Check sheet for the modelled part. Datum: model origin and axes. Units: mm. Coordinates: 2 decimals unless noted, no trailing zeros. Loops run counter-clockwise (first coordinate to the right, second up) from the corner with the lowest first, then second, coordinate; pieces in that order, holes last. Notation, with made-up numbers: (28.25, -13) -> (57.25, -13) arc R10 ccw to (57.25, 0) -> close; hole circle Ø9 at (19, -30). An arc over 180 degrees is marked (long way). Use CSV: the item, a comma, the result in double quotes.
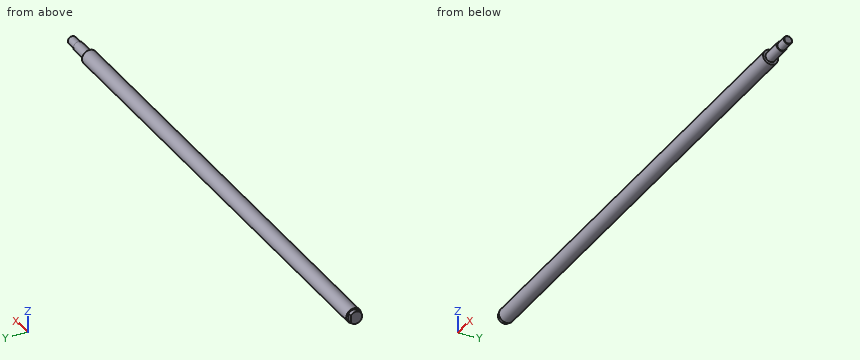
```python
from build123d import *

# Parameters (mm, degrees)
CHAMFER1_SIZE       = 0.5
BOSS_EXTRUDE1_DEPTH = 5


with BuildPart() as part:
    # Sketch1 → Revolve1 (revolve)
    with BuildSketch(Plane.XY, mode=Mode.PRIVATE) as revolve1_sk:
        Polygon((0, 0), (-640, 0), (-640, 9), (-40, 9), (-40, 6), (-15, 6), (-15, 5), (0, 5), align=None)
    revolve(revolve1_sk.sketch.rotate(Axis((-640, 0, 0), (1, 0, 0)), 90), axis=Axis((-640, 0, 0), (1, 0, 0)))

    # Chamfer1
    chamfer1_edges = [part.edges().sort_by_distance(p)[0] for p in [
        (0, 0, -5),
    ]]
    chamfer(chamfer1_edges, length=CHAMFER1_SIZE)

    # Sketch2 → Boss-Extrude1 (add)
    with BuildSketch(Plane.ZY.offset(640)):
        with BuildLine():
            Line((-4.485716723, 6.010685941), (4.485716723, 6.010685941))
            ThreePointArc((4.485716723, 6.010685941), (0, -7.5), (-4.485716723, 6.010685941))
        make_face()
    extrude(amount=BOSS_EXTRUDE1_DEPTH)


solid = part.part
```
1) Go/stop test with flat-tipped pins: pin 1 Ø8 at (x, z) = (-353, 2.5) entering from +Y; pin 2 Ø1.5 at (x, z) = (-355, 3.5) entering from +Y; pin 3 Ø5 at (y, z) = (-7, -3) entering from +X; pin 4 Ø6 at (x, z) = (-177.5, -7) entering from +Y. Record where each tip stops, or that it passes through.
Answer below:
pin 1,"stops at y = 9"
pin 2,"stops at y = 8.57"
pin 3,"stops at x = -15"
pin 4,"stops at y = 8.06"
2) Thickness scan on line 1 along X through (y, z) = (-5.25, 2.5); line 2 along Z through (x, y) = (-268, 7.5); line 3 along Z through (x, y) = (-128.5, 1). Record the ranges inside material, lowest first. Write a range as from..to.
Answer below:
line 1,"x = -645..-15"
line 2,"z = -4.97..4.97"
line 3,"z = -8.94..8.94"
3) Cross-section at C-C on x = -345. Record the boundary of the cut face in (y, z), and give its area (3 significant figures).
Answer below:
outline,"circle Ø18 at (0, 0)"
area,"254 mm²"
4) Cross-section at A-A on z = 0. Record the boundary of the cut face in (x, y).
Answer below:
outline,"(-645, -7.5) -> (-640, -7.5) -> (-640, -9) -> (-40, -9) -> (-40, -6) -> (-15, -6) -> (-15, -5) -> (-0.5, -5) -> (0, -4.5) -> (0, 4.5) -> (-0.5, 5) -> (-15, 5) -> (-15, 6) -> (-40, 6) -> (-40, 9) -> (-640, 9) -> (-640, 6.01) -> (-645, 6.01) -> close"
5) Cross-section at B-B on y = 0. Record the boundary of the cut face in (x, z).
Answer below:
outline,"(-645, -7.5) -> (-640, -7.5) -> (-640, -9) -> (-40, -9) -> (-40, -6) -> (-15, -6) -> (-15, -5) -> (-0.5, -5) -> (0, -4.5) -> (0, 4.5) -> (-0.5, 5) -> (-15, 5) -> (-15, 6) -> (-40, 6) -> (-40, 9) -> (-640, 9) -> (-640, 7.5) -> (-645, 7.5) -> close"
